Autodesk Inventor part; units mm, degrees
ref_plane "YZ Plane" through (0, 0, 0) normal (1, 0, 0) x (0, 1, 0)
ref_plane "XZ Plane" through (0, 0, 0) normal (0, 1, 0) x (-1, 0, 0)
ref_plane "XY Plane" through (0, 0, 0) normal (0, 0, 1) x (1, 0, 0)
sketch "Sketch1" plane through (0, 0, 0) normal (0, 0, 1) x (1, 0, 0)
  arc A0 (0, 0) -> (0, -7) centre (0, -3.5) ccw
  circle A1 centre (0, -3.5) radius 2.5
  circle A2 centre (0, -3.5) radius 3
  circle A3 centre (32, -3.5) radius 2.5
  circle A4 centre (32, -3.5) radius 3
  circle A5 centre (8, -3.5) radius 2.5
  circle A6 centre (8, -3.5) radius 3
  circle A7 centre (16, -3.5) radius 3
  circle A8 centre (16, -3.5) radius 2.5
  circle A9 centre (24, -3.5) radius 3
  circle A10 centre (24, -3.5) radius 2.5
  circle A11 centre (32, -19.5) radius 3
  circle A12 centre (32, -19.5) radius 2.5
  line L0 (28.5, -19.5) -> (28.5, -7)
  line L1 (35.5, -19.5) -> (35.5, -7)
  circle A13 centre (32, -11.5) radius 2.5
  circle A14 centre (32, -11.5) radius 3
  arc A15 (28.5, -19.5) -> (35.5, -19.5) centre (32, -19.5) ccw
  line L2 (35.5, -7) -> (35.5, 0)
  line L3 (0, -7) -> (28.5, -7)
  line L4 (0, 0) -> (35.5, 0)
extrude "Extrusion1" add sketch "Sketch1" along normal blind 8 contours L4 L2 L1 A15 L0 L3 A0 | A2 | A4 | A6 | A7 | A9 | A11 | A14
extrude "Extrusion2" cut sketch "Sketch1" along normal blind 1 contours A2 | A4 | A6 | A7 | A9 | A11 | A14
sketch "Sketch2" plane through (0, 0, 8) normal (0, 0, 1) x (1, 0, 0)
  circle A0 centre (32, -11.5) radius 2.5
  circle A1 centre (32, -19.5) radius 2.5
  circle A2 centre (24, -3.5) radius 2.5
  circle A3 centre (16, -3.5) radius 2.5
  circle A4 centre (8, -3.5) radius 2.5
  circle A5 centre (32, -3.5) radius 2.5
  circle A6 centre (0, -3.5) radius 2.5
  circle A7 centre (0, -3.5) radius 3
  circle A8 centre (8, -3.5) radius 3
  circle A9 centre (16, -3.5) radius 3
  circle A10 centre (24, -3.5) radius 3
  circle A11 centre (32, -3.5) radius 3
  circle A12 centre (32, -11.5) radius 3
  circle A13 centre (32, -19.5) radius 3
extrude "Extrusion3" cut sketch "Sketch2" against normal blind 1
fillet "Fillet1" radius 2 1 edges at (35.5, 0, 4)
fillet "Fillet2" radius 2 1 edges at (28.5, -7, 4)
properties part number "technic L 5 barrenos"
CAD build for the part. Positions are in the model's coordinates, mm. A direction names the side the tool comes from. Give positions to 0.01 mm unless a question says otherwise; leave off trailing zeros. Order: outer loops, then holes, each group sorted by start corner. A loop starts at its lowest first (then second) coordinate and runs counter-clockwise, first axis right, second up.
(1) Tool access for faces 1 (the cylindrical face through (29.6, -21.3, 7.5)), 2 (the cylindrical face through (21, -3.6, 0.5)), 3 (the cylindrical face through (0, -6, 4)): list every direction of +Z, -Z, +X, -X, +Y, -Y with a clear straight run to the whole face (end or side of a thin tool).
(2) Saw through at B-B, the plane y = -11.5. Give the cut face in (x, z), then the cut area to 3 significant figures.
(3) Saw through at D-D, the plane x = 32. State how many separate pieces and enclosed holes the cut face has, then the cut area to 3 significant figures.
(4) Flat gauge pins, fed straight in: pin 1 (3.5 mm diameter, centred on x = 8, y = -3.5, fed in from -Z); pin 2 (1.5 mm diameter, centred on y = -10.5, z = 3, fed in from -X); pin 3 (3 mm diameter, centred on x = 33, y = -4.5, fed in from -Z); pin 4 (5.5 mm diameter, centred on x = 24, y = -3.5, fed in from +Z). Where does each tip first touch, or does it go through?
(5) Saw through at C-C, the plane x = 8. Give the cut face in (y, z), then the cut area to 3 significant figures.
(6) Saw through at A-A, the plane z = 3.25. Give the cut face in (x, y).
(7) Mould opens along Y. For faces 4 (the cylindrical face through (32, -23, 4)), 5 (the flat face through (35.5, -11, 4)), 6 (the flat face through (31, -9, 7)) say: released by +Y, released by -Y, zero draft, split by the parting line, or undercut.
(8) Drill centre lines: L1, parallel to Y at x = 24, z = 0.65; L2, parallel to Y at x = 0, z = 3; L3, parallel to Y at x = 3.5, z = 4. Where is each one in solid material? Low to high.
Results found:
1. face 1: +Z
1. face 2: -Z
1. face 3: +Z, -Z
2. outline: (28.5, 0) - (29, 0) - (29, 1) - (29.5, 1) - (29.5, 7) - (29, 7) - (29, 8) - (28.5, 8) - close; (34.5, 1) - (35, 1) - (35, 0) - (35.5, 0) - (35.5, 8) - (35, 8) - (35, 7) - (34.5, 7) - close
2. area: 14.0 mm2
3. separate pieces: 4
3. enclosed holes: 0
3. area: 58.0 mm2
4. pin 1: passes through
4. pin 2: stops at x = 28.5
4. pin 3: stops at z = 1
4. pin 4: stops at z = 7
5. outline: (-7, 0) - (-6.5, 0) - (-6.5, 1) - (-6, 1) - (-6, 7) - (-6.5, 7) - (-6.5, 8) - (-7, 8) - close; (-1, 1) - (-0.5, 1) - (-0.5, 0) - (0, 0) - (0, 8) - (-0.5, 8) - (-0.5, 7) - (-1, 7) - close
5. area: 14.0 mm2
6. outline: (0, -7) - (26.5, -7) arc R2 cw to (28.5, -9) - (28.5, -19.5) arc R3.5 ccw to (35.5, -19.5) - (35.5, -2) arc R2 ccw to (33.5, 0) - (0, 0) arc R3.5 ccw to start; hole circle Ø5 at (0, -3.5); hole circle Ø5 at (8, -3.5); hole circle Ø5 at (16, -3.5); hole circle Ø5 at (24, -3.5); hole circle Ø5 at (32, -19.5); hole circle Ø5 at (32, -11.5); hole circle Ø5 at (32, -3.5)
7. face 4: released by -Y
7. face 5: zero draft
7. face 6: undercut
8. L1: y = -7 to -6.5, -0.5 to 0
8. L2: y = -7 to -6, -1 to 0
8. L3: y = -7 to 0
